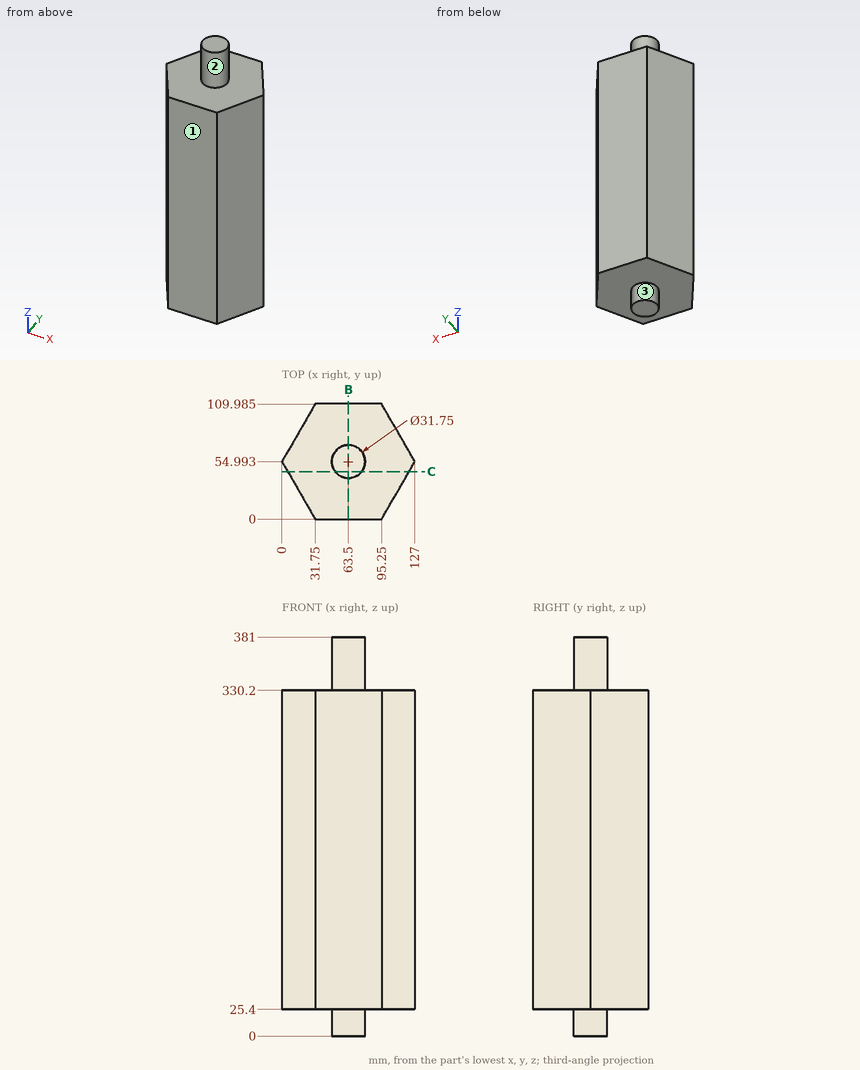
Print and shaded views of the part. All mm, measured from the part's lowest x, y and z. A direction names the side the tool comes from. Coordinates: 2 decimals unless noted, no trailing zeros. Loops run counter-clockwise (first coordinate to the right, second up) from the corner with the lowest first, then second, coordinate; pieces in that order, holes last. Notation, with made-up numbers: M 37.5,-30.5 L 82.5,-30.5 A35 cw 82.5,4.5 Z; hole C -28.75,25 d7. An arc over 180 degrees is marked long. Use a Markdown table: item, result. Add a question column.
Q1. Cut at B-B (x = 63.5). Write the cut outline in (y, z) (1 decimal).
Q2. Pin check, flat tips, straight feed: P1, Ø3, axis at y = 52.5, z = 95, coming from the -X side; P2, Ø5, axis at x = 85.5, y = 65.5, coming from the -Z side; P3, Ø4, axis at y = 31.5, z = 90, coming from the +X side. Stop position of each tip, or through.
Q3. Which spindle directions (+Z, -Z, +X, -X, +Y, -Y) get a long thin tool onto all of the face, cutting with end or side? Do the marked faces 1, 2 and 3. Say none if no direction does.
Q4. Cut at C-C (y = 45.5). Write the cut outline in (x, z) (1 decimal).
Q5. Probe L1, parallel to X at y = 54.5, z = 366; L2, parallel to Z at x = 100, y = 100.5; L3, parallel to X at y = 46, z = 32.5. List the from-to ranges inside material, lowest first.
Worked out:
| question | item | result |
|---|---|---|
| 1 | outline | M 0,25.4 L 39.1,25.4 L 39.1,0 L 70.9,0 L 70.9,25.4 L 110,25.4 L 110,330.2 L 70.9,330.2 L 70.9,381 L 39.1,381 L 39.1,330.2 L 0,330.2 Z |
| 2 | P1 | stops at x = 0.57 |
| 2 | P2 | stops at z = 25.4 |
| 2 | P3 | stops at x = 114.59 |
| 3 | face 1 | +Z, -Z, +X, -X, -Y |
| 3 | face 2 | +Z |
| 3 | face 3 | -Z |
| 4 | outline | M 5.5,25.4 L 50.8,25.4 L 50.8,0 L 76.2,0 L 76.2,25.4 L 121.5,25.4 L 121.5,330.2 L 76.2,330.2 L 76.2,381 L 50.8,381 L 50.8,330.2 L 5.5,330.2 Z |
| 5 | L1 | x = 47.63 to 79.37 |
| 5 | L2 | z = 25.4 to 330.2 |
| 5 | L3 | x = 5.19 to 121.81 |
